Design review of the part built by this model. Coordinates are the model's own, in mm. Face numbers are marked on the shaded views. A direction names the side the tool comes from. Coordinates: 2 decimals unless noted, no trailing zeros. Loops run counter-clockwise (first coordinate to the right, second up) from the corner with the lowest first, then second, coordinate; pieces in that order, holes last. Notation, with made-up numbers: (55, 78.25) - (72, 78.25) arc R34 cw to (72, 116.25) - close; hole circle Ø5 at (-7.5, 46). An arc over 180 degrees is marked (long way). Answer in a Markdown table with one row per item. Add a question column.
(1) We need section B-B, the plane x = 87.5. Write out the cut boundary in (y, z).
(2) Clearance check with flat-ended pins moving along their axes: pin 1 (12 mm diameter, centred on x = 115, y = -2, fed in from +Z); pin 2 (3.5 mm diameter, centred on y = 0, z = 0, fed in from -X); pin 3 (2 mm diameter, centred on x = 8.5, y = -1, fed in from +Z). State where each tip first meets the part, or that it passes through.
(3) We need section A-A, the plane x = 19.5. Write out the cut boundary in (y, z), plus the area to 3 significant figures.
(4) For the marked faces 1, 2, 3 and 4, list the 3-axis set-ups (+Z, -Z, +X, -X, +Y, -Y) from which the entire face can be reached by the end or side of a thin tool; tool diameter is ignored.
(5) To check wall thickness, follow L1, parallel to Y at x = 6.5, z = 0; L2, parallel to Y at x = 136.15, z = 0; L3, parallel to Z at x = 28.5, y = -4. State the ranges of each line that lie inside material, in increasing order. Write a range as [from, to].
from build123d import *

# Parameters (mm, degrees)
EXTRUDE_1_DEPTH     = 15
M5X0_8_1_D          = 4.2
M5X0_8_1_DEPTH      = 12.4
M5X0_8_1_TIP        = 1.2618073
SKETCH_5_R          = 7.5
EXTRUDE_2_DEPTH     = 15
SKETCH_6_R          = 10.5
EXTRUDE_3_DEPTH     = 30
SKETCH_7_R          = 12.5
EXTRUDE_4_DEPTH     = 23
SKETCH_8_R          = 10.5
EXTRUDE_5_DEPTH     = 30
CHAMFER_1_SIZE      = 1
CHAMFER_2_SIZE      = 1
SKETCH_9_R          = 7.5
EXTRUDE_6_DEPTH     = 25
CHAMFER_3_SIZE      = 1
SKETCH_10_R         = 3.5
CUT_EXTRUDE_1_DEPTH = 2.5
CHAMFER_4_SIZE      = 0.5


with BuildPart() as part:
    # 草图1 → 凸台-拉伸1 (new body)
    with BuildSketch(Plane(origin=(0, 0, 0), x_dir=(0, 0, -1), z_dir=(1, 0, 0))):
        Polygon((0, -7.332348419), (6.35, -3.666174209), (6.35, 3.666174209), (0, 7.332348419), (-6.35, 3.666174209), (-6.35, -3.666174209), align=None)
    extrude(amount=EXTRUDE_1_DEPTH)

    # M5x0.8 螺纹孔1
    with Locations(Plane.ZY):
        with Locations((0, 0)):
            Hole(M5X0_8_1_D / 2, depth=M5X0_8_1_DEPTH)
            with Locations((0, 0, -(M5X0_8_1_DEPTH + M5X0_8_1_TIP / 2))):  # 118° drill point
                Cone(0, M5X0_8_1_D / 2, M5X0_8_1_TIP, mode=Mode.SUBTRACT)

    # 草图5 → 凸台-拉伸2 (add)
    with BuildSketch(Plane(origin=(15, 0, 0), x_dir=(0, 0, -1), z_dir=(1, 0, 0))):
        Circle(SKETCH_5_R)
    extrude(amount=EXTRUDE_2_DEPTH)

    # 草图6 → 凸台-拉伸3 (add)
    with BuildSketch(Plane(origin=(30, 0, 0), x_dir=(0, 0, -1), z_dir=(1, 0, 0))):
        Circle(SKETCH_6_R)
    extrude(amount=EXTRUDE_3_DEPTH)

    # 草图7 → 凸台-拉伸4 (add)
    with BuildSketch(Plane(origin=(60, 0, 0), x_dir=(0, 0, -1), z_dir=(1, 0, 0))):
        Circle(SKETCH_7_R)
    extrude(amount=EXTRUDE_4_DEPTH)

    # 草图8 → 凸台-拉伸5 (add)
    with BuildSketch(Plane(origin=(83, 0, 0), x_dir=(0, 0, -1), z_dir=(1, 0, 0))):
        Circle(SKETCH_8_R)
    extrude(amount=EXTRUDE_5_DEPTH)

    # 倒角1
    chamfer_1_edges = [part.edges().sort_by_distance(p)[0] for p in [
        (30, 0, 10.5),
    ]]
    chamfer(chamfer_1_edges, length=CHAMFER_1_SIZE)

    # 倒角2
    chamfer_2_edges = [part.edges().sort_by_distance(p)[0] for p in [
        (113, 0, 10.5),
    ]]
    chamfer(chamfer_2_edges, length=CHAMFER_2_SIZE)

    # 草图9 → 凸台-拉伸6 (add)
    with BuildSketch(Plane(origin=(113, 0, 0), x_dir=(0, 0, -1), z_dir=(1, 0, 0))):
        Circle(SKETCH_9_R)
    extrude(amount=EXTRUDE_6_DEPTH)

    # 倒角3
    chamfer_3_edges = [part.edges().sort_by_distance(p)[0] for p in [
        (138, 0, 7.5),
    ]]
    chamfer(chamfer_3_edges, length=CHAMFER_3_SIZE)

    # 草图10 → 切除-拉伸1 (cut)
    with BuildSketch(Plane(origin=(138, 0, 0), x_dir=(0, 0, -1), z_dir=(1, 0, 0))):
        Circle(SKETCH_10_R)
    extrude(amount=-CUT_EXTRUDE_1_DEPTH, mode=Mode.SUBTRACT)

    # 倒角4
    chamfer_4_edges = [part.edges().sort_by_distance(p)[0] for p in [
        (138, 0, 3.5),
    ]]
    chamfer(chamfer_4_edges, length=CHAMFER_4_SIZE)


solid = part.part
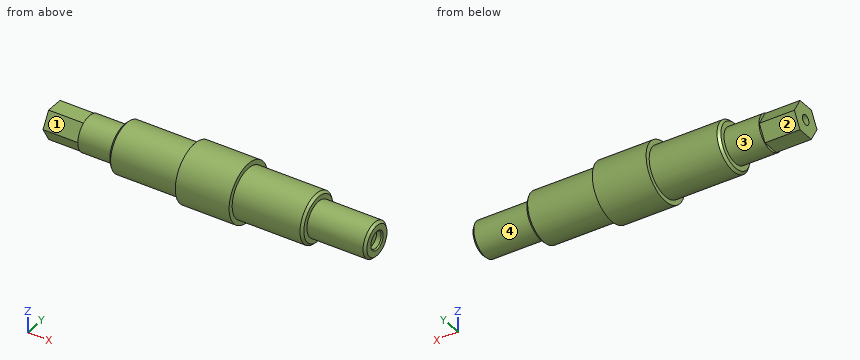
Responses:
| question | item | result |
|---|---|---|
| 1 | outline | circle Ø21 at (0, 0) |
| 2 | pin 1 | stops at z = 10.5 |
| 2 | pin 2 | stops at x = 12.61 |
| 2 | pin 3 | stops at z = 6.35 |
| 3 | outline | circle Ø15 at (0, 0) |
| 3 | area | 177 mm2 |
| 4 | face 1 | +Z, -X, -Y |
| 4 | face 2 | -Z, -X, +Y |
| 4 | face 3 | -X |
| 4 | face 4 | +X |
| 5 | L1 | y = [-7.33, -2.1], [2.1, 7.33] |
| 5 | L2 | y = [-7.5, -3.5], [3.5, 7.5] |
| 5 | L3 | z = [-6.34, 6.34] |
